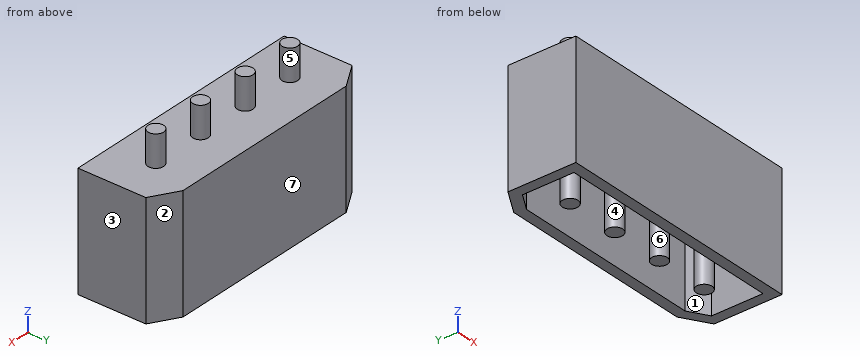
```python
from build123d import *

# Parameters (mm, degrees)
EXTRUDE_1_DEPTH        = 11
CUT_EXTRUDE_1_DEPTH    = 9
SKETCH_3_R             = 0.75
EXTRUDE_2_DEPTH        = 9
SKETCH_4_R             = 1.77312928
CUT_EXTRUDE_2_DEPTH    = 4
PATTERN_LINEAR_1_COUNT = 4
PATTERN_LINEAR_1_PITCH = 5.2


with BuildPart() as part:
    # 草图1 → 凸台-拉伸1 (new body)
    with BuildSketch(Plane.XY):
        Polygon((0, 0), (-24, 0), (-24, 6.5), (-21.5, 8), (-2.5, 8), (0, 6.5), align=None)
    extrude(amount=EXTRUDE_1_DEPTH)

    # 草图2 → 切除-拉伸1 (cut)
    with BuildSketch(Plane(origin=(0, 0, 0), x_dir=(-1, 0, 0), z_dir=(0, 0, -1))):
        Polygon((1, 5.933809621), (1, 1), (23, 1), (23, 5.933809621), (21.223016035, 7), (2.776983965, 7), align=None)
    extrude(amount=-CUT_EXTRUDE_1_DEPTH, mode=Mode.SUBTRACT)

    # 草图3 → 凸台-拉伸2 (add, symmetric)
    with BuildSketch(Plane(origin=(0, 0, 9), x_dir=(-1, 0, 0), z_dir=(0, 0, -1))):
        with Locations(Location((4.2, 4, 0), (0, 0, 180))):
            Circle(SKETCH_3_R)
    extrude_2 = extrude(amount=EXTRUDE_2_DEPTH, both=True)

    # 草图4 → 切除-拉伸2 (cut)
    with BuildSketch(Plane.XY.offset(18)):
        with Locations((-4.2, 4)):
            Circle(SKETCH_4_R)
    cut_extrude_2 = extrude(amount=-CUT_EXTRUDE_2_DEPTH, mode=Mode.SUBTRACT)

    # 阵列(线性)1: 凸台-拉伸2, 切除-拉伸2 ×4
    with Locations(*[(-i * PATTERN_LINEAR_1_PITCH, 0, 0) for i in range(1, PATTERN_LINEAR_1_COUNT)]):
        add(extrude_2)
        add(cut_extrude_2, mode=Mode.SUBTRACT)


solid = part.part
```
Check sheet for the modelled part. Datum: model origin and axes. Units: mm. Face numbers are marked on the shaded views. A direction names the side the tool comes from. Round coordinates to 2 decimals unless told otherwise and drop trailing zeros. Loops run counter-clockwise (first coordinate to the right, second up) from the corner with the lowest first, then second, coordinate; pieces in that order, holes last. Notation, with made-up numbers: M 50,-14.5 L 71,-14.5 A21 cw 71,7.5 Z; hole C 81,82 d9. An arc over 180 degrees is marked long. Answer as a JSON object with one key per item and string values.
1. Gauge pin test, flat end, axial feed: P1, Ø1, axis at x = -18.5, y = 1.5, coming from the +Z side. Record the tip position at first contact, or that the pin passes through.
Reply:
{"P1": "stops at z = 11"}
2. Scan lines: line 1 (Y direction, x = -14.5, z = 4.75); line 2 (Y direction, x = -8.25, z = 5.5); line 3 (X direction, y = 4.5, z = 13). Record each from-to range of solid material in increasing order.
Reply:
{"line 1": "y = 0 to 1, 3.26 to 4.74, 7 to 8", "line 2": "y = 0 to 1, 7 to 8", "line 3": "x = -20.36 to -19.24, -15.16 to -14.04, -9.96 to -8.84, -4.76 to -3.64"}
3. Section check D-D (x = -17.75). Record the boundary of the cut face in (y, z).
Reply:
{"outline": "M 0,0 L 1,0 L 1,9 L 7,9 L 7,0 L 8,0 L 8,11 L 0,11 Z"}
4. Access from +Z, -Z, +X, -X, +Y, -Y to the whole of each face (thin tool, end or side, straight path). Record for the marked faces 5, 6 and 7.
Reply:
{"face 5": "+Z", "face 6": "-Z", "face 7": "+Z, -Z, +X, -X, +Y"}
5. Section check C-C (x = -9.4). Record the boundary of the cut face in (y, z).
Reply:
{"outline": "M 0,0 L 1,0 L 1,9 L 3.25,9 L 3.25,0 L 4.75,0 L 4.75,9 L 7,9 L 7,0 L 8,0 L 8,11 L 4.75,11 L 4.75,14 L 3.25,14 L 3.25,11 L 0,11 Z"}
6. Section check A-A (z = 1). Record the boundary of the cut face in (x, y), plus the area to 3 significant figures.
Reply:
{"outline": "M -24,0 L 0,0 L 0,6.5 L -2.5,8 L -21.5,8 L -24,6.5 Z; C -19.8,4 d1.5; C -14.6,4 d1.5; C -9.4,4 d1.5; C -4.2,4 d1.5; hole M -23,1 L -1,1 L -1,5.93 L -2.78,7 L -21.22,7 L -23,5.93 Z", "area": "65.2 mm²"}
7. Section check B-B (y = 5). Record the boundary of the cut face in (x, z).
Reply:
{"outline": "M -24,0 L -23,0 L -23,9 L -1,9 L -1,0 L 0,0 L 0,11 L -24,11 Z"}
8. Mould release check, pull along Y, two halves, no side actions. Record for the marked faces 1, 2, 3 and 4: pulls with the +Y half, pulls with the -Y half, needs draft (parallel to the pull), parting line crosses it, or undercut.
Reply:
{"face 1": "undercut", "face 2": "pulls with the +Y half", "face 3": "needs draft", "face 4": "undercut"}
